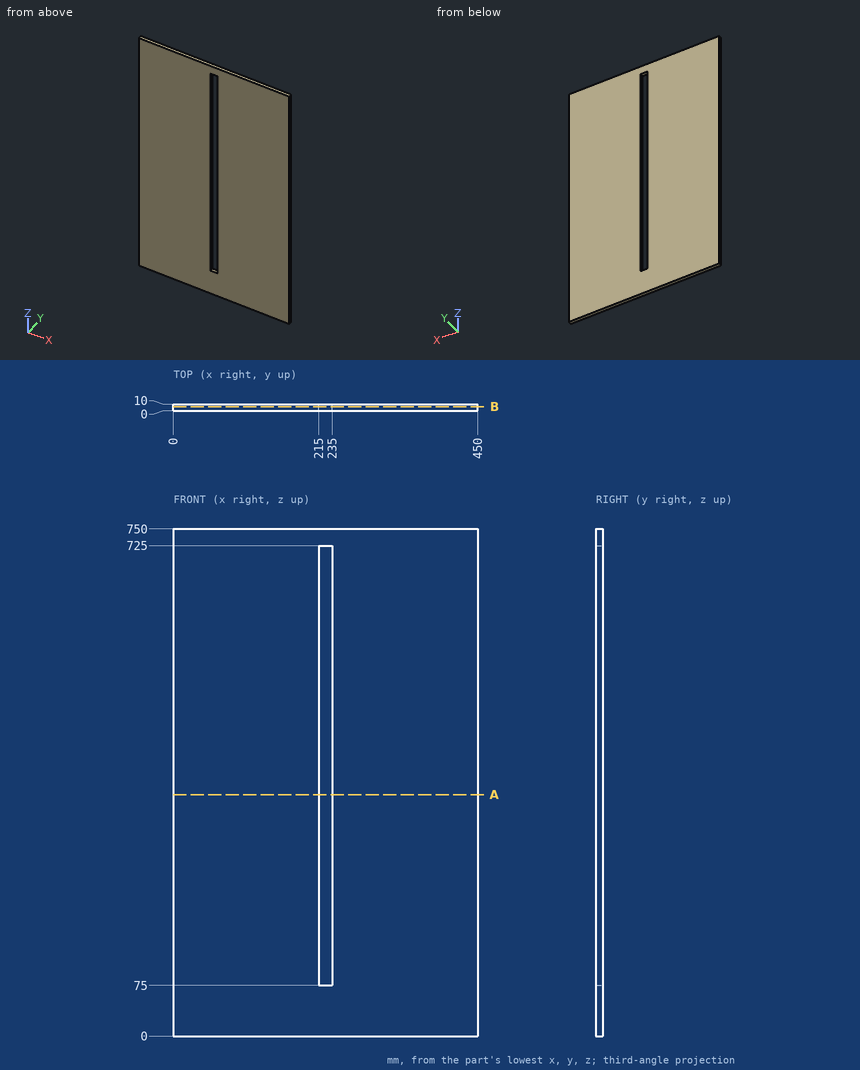
Input: dimensioned drawing with shaded views. Units: mm. Origin: part minimum x, y, z. Coordinates: 2 decimals unless noted, no trailing zeros. Order: outer loops, then holes, each group sorted by start corner. A loop starts at its lowest first (then second) coordinate and runs counter-clockwise, first axis right, second up. Notation, with made-up numbers: (-3.75, 24.25) -> (45.25, 24.25) arc R22 ccw to (45.25, 59.25) -> close; hole circle Ø2 at (-7, 41). An arc over 180 degrees is marked (long way). Answer in a Markdown table with one row per item.
Item 1: Ray query, L1, parallel to X at y = 5, z = 674; L2, parallel to Z at x = 230.5, y = 8.75. Return the intervals inside material, ascending.
Return value:
| item | result |
|---|---|
| L1 | x = 0 to 215, 235 to 450 |
| L2 | z = 0 to 75, 725 to 750 |
Item 2: Section B-B on y = 6. Output: boundary loops of the cut face in (x, z), plus the area to 4 significant figures.
Return value:
| item | result |
|---|---|
| outline | (0, 0) -> (450, 0) -> (450, 750) -> (0, 750) -> close; hole (215, 75) -> (235, 75) -> (235, 725) -> (215, 725) -> close |
| area | 324,500 mm² |
Item 3: Section A-A on z = 357. Output: boundary loops of the cut face in (x, y).
Return value:
| item | result |
|---|---|
| outline | (0, 0) -> (215, 0) -> (215, 10) -> (0, 10) -> close; (235, 0) -> (450, 0) -> (450, 10) -> (235, 10) -> close |
